from build123d import *

# Parameters (mm, degrees)
SKETCH2_R                             = 14
SKETCH2_R_2                           = 8
BOSS_EXTRUDE7_DEPTH                   = 15
SKETCH2_9_R                           = 16
SKETCH2_9_R_2                         = 13
BOSS_EXTRUDE8_DEPTH                   = 15
SKETCH2_11_R                          = 13
SKETCH2_11_R_2                        = 10
BOSS_EXTRUDE9_DEPTH                   = 9.5
BOSS_EXTRUDE11_REACH                  = 219.372
BOSS_EXTRUDE11_END_RADIUS             = 14
BOSS_EXTRUDE11_DIRECTION_2_REACH      = 219.372
BOSS_EXTRUDE11_DIRECTION_2_END_RADIUS = 16
BOSS_EXTRUDE12_REACH                  = 219.489
SKETCH15_W                            = 3
SKETCH15_H                            = 9.5
FILLET1_R                             = 2
SKETCH2_13_R                          = 8
SKETCH2_13_R_2                        = 4.25
BOSS_EXTRUDE13_DEPTH                  = 11


with BuildPart() as part:
    # Sketch2 → Boss-Extrude7 (new body)
    with BuildSketch(Plane(origin=(0, 0, 0), x_dir=(1, 0, 0), z_dir=(0, 1, 0))):
        with Locations(Location((-50, 3.220631283, 0), (0, 0, 270))):
            Circle(SKETCH2_R)
        with Locations(Location((-50, 3.220631283, 0), (0, 0, 270))):
            Circle(SKETCH2_R_2, mode=Mode.SUBTRACT)
    extrude(amount=BOSS_EXTRUDE7_DEPTH)


with BuildPart() as body_2:
    # Sketch2<9> → Boss-Extrude8 (new body)
    with BuildSketch(Plane(origin=(0, 0, 0), x_dir=(1, 0, 0), z_dir=(0, 1, 0))):
        with Locations(Location((200, 3.220631283, 0), (0, 0, 270))):
            Circle(SKETCH2_9_R)
        with Locations(Location((200, 3.220631283, 0), (0, 0, 270))):
            Circle(SKETCH2_9_R_2, mode=Mode.SUBTRACT)
    extrude(amount=BOSS_EXTRUDE8_DEPTH)

    # Sketch2<11> → Boss-Extrude9 (add)
    with BuildSketch(Plane(origin=(0, 0, 0), x_dir=(1, 0, 0), z_dir=(0, 1, 0))):
        with Locations(Location((200, 3.220631283, 0), (0, 0, 270))):
            Circle(SKETCH2_11_R)
        with Locations(Location((200, 3.220631283, 0), (0, 0, 270))):
            Circle(SKETCH2_11_R_2, mode=Mode.SUBTRACT)
    extrude(amount=BOSS_EXTRUDE9_DEPTH)


    add(part.part)  # Boss-Extrude11 merges part
    # Boss-Extrude11: up to this cylinder (the profile starts outside it)
    boss_extrude11_end = Plane(origin=(-50, 0.212132, -3.220631283), z_dir=(0, -1, 0)) * Cylinder(BOSS_EXTRUDE11_END_RADIUS, 467.744, mode=Mode.PRIVATE)
    # Sketch3 → Boss-Extrude11 (add, up to the surface)
    with BuildSketch(Plane(origin=(0, 0, 0), x_dir=(0, 0, -1), z_dir=(1, 0, 0)), mode=Mode.PRIVATE) as boss_extrude11_sk1:
        Polygon((10.720631283, 0), (10.720631283, 15), (-4.279368717, 15), (-4.279368717, 0), (-1.279368717, 0), (-1.279368717, 12), (7.720631283, 12), (7.720631283, 0), align=None)
    boss_extrude11_tool1 = extrude(boss_extrude11_sk1.sketch, amount=-BOSS_EXTRUDE11_REACH, mode=Mode.PRIVATE) - boss_extrude11_end
    add(boss_extrude11_tool1.solids().sort_by_distance((0, 0.212132, -9.220631))[0])

    # Boss-Extrude11 direction 2: up to this cylinder (the profile starts outside it)
    boss_extrude11_direction_2_end = Plane(origin=(200, 0.212132, -3.220631283), z_dir=(0, -1, 0)) * Cylinder(BOSS_EXTRUDE11_DIRECTION_2_END_RADIUS, 471.744, mode=Mode.PRIVATE)
    # Sketch3 → Boss-Extrude11 direction 2 (add, up to the surface)
    with BuildSketch(Plane(origin=(0, 0, 0), x_dir=(0, 0, -1), z_dir=(1, 0, 0)), mode=Mode.PRIVATE) as boss_extrude11_direction_2_sk1:
        Polygon((10.720631283, 0), (10.720631283, 15), (-4.279368717, 15), (-4.279368717, 0), (-1.279368717, 0), (-1.279368717, 12), (7.720631283, 12), (7.720631283, 0), align=None)
    boss_extrude11_direction_2_tool1 = extrude(boss_extrude11_direction_2_sk1.sketch, amount=BOSS_EXTRUDE11_DIRECTION_2_REACH, mode=Mode.PRIVATE) - boss_extrude11_direction_2_end
    add(boss_extrude11_direction_2_tool1.solids().sort_by_distance((0, 0.212132, -9.220631))[0])

    # Sketch15 → Boss-Extrude12 (add, up to next)
    with BuildSketch(Plane.XY.offset(-7.720631283), mode=Mode.PRIVATE) as boss_extrude12_sk1:
        with Locations((-14.45117452, 7.25)):
            Rectangle(SKETCH15_W, SKETCH15_H)
    boss_extrude12_tool1 = extrude(boss_extrude12_sk1.sketch, amount=BOSS_EXTRUDE12_REACH, mode=Mode.PRIVATE) - body_2.part
    # Sketch15 → Boss-Extrude12 (add, up to next)
    with BuildSketch(Plane.XY.offset(-7.720631283), mode=Mode.PRIVATE) as boss_extrude12_sk2:
        with Locations((86.457765729, 7.25)):
            Rectangle(SKETCH15_W, SKETCH15_H)
    boss_extrude12_tool2 = extrude(boss_extrude12_sk2.sketch, amount=BOSS_EXTRUDE12_REACH, mode=Mode.PRIVATE) - body_2.part
    # Sketch15 → Boss-Extrude12 (add, up to next)
    with BuildSketch(Plane.XY.offset(-7.720631283), mode=Mode.PRIVATE) as boss_extrude12_sk3:
        with Locations((10.776060542, 7.25)):
            Rectangle(SKETCH15_W, SKETCH15_H)
    boss_extrude12_tool3 = extrude(boss_extrude12_sk3.sketch, amount=BOSS_EXTRUDE12_REACH, mode=Mode.PRIVATE) - body_2.part
    # Sketch15 → Boss-Extrude12 (add, up to next)
    with BuildSketch(Plane.XY.offset(-7.720631283), mode=Mode.PRIVATE) as boss_extrude12_sk4:
        with Locations((36.003295604, 7.25)):
            Rectangle(SKETCH15_W, SKETCH15_H)
    boss_extrude12_tool4 = extrude(boss_extrude12_sk4.sketch, amount=BOSS_EXTRUDE12_REACH, mode=Mode.PRIVATE) - body_2.part
    # Sketch15 → Boss-Extrude12 (add, up to next)
    with BuildSketch(Plane.XY.offset(-7.720631283), mode=Mode.PRIVATE) as boss_extrude12_sk5:
        with Locations((61.230530666, 7.25)):
            Rectangle(SKETCH15_W, SKETCH15_H)
    boss_extrude12_tool5 = extrude(boss_extrude12_sk5.sketch, amount=BOSS_EXTRUDE12_REACH, mode=Mode.PRIVATE) - body_2.part
    # Sketch15 → Boss-Extrude12 (add, up to next)
    with BuildSketch(Plane.XY.offset(-7.720631283), mode=Mode.PRIVATE) as boss_extrude12_sk6:
        with Locations((111.685000791, 7.25)):
            Rectangle(SKETCH15_W, SKETCH15_H)
    boss_extrude12_tool6 = extrude(boss_extrude12_sk6.sketch, amount=BOSS_EXTRUDE12_REACH, mode=Mode.PRIVATE) - body_2.part
    # Sketch15 → Boss-Extrude12 (add, up to next)
    with BuildSketch(Plane.XY.offset(-7.720631283), mode=Mode.PRIVATE) as boss_extrude12_sk7:
        with Locations((136.912235853, 7.25)):
            Rectangle(SKETCH15_W, SKETCH15_H)
    boss_extrude12_tool7 = extrude(boss_extrude12_sk7.sketch, amount=BOSS_EXTRUDE12_REACH, mode=Mode.PRIVATE) - body_2.part
    # Sketch15 → Boss-Extrude12 (add, up to next)
    with BuildSketch(Plane.XY.offset(-7.720631283), mode=Mode.PRIVATE) as boss_extrude12_sk8:
        with Locations((162.139470915, 7.25)):
            Rectangle(SKETCH15_W, SKETCH15_H)
    boss_extrude12_tool8 = extrude(boss_extrude12_sk8.sketch, amount=BOSS_EXTRUDE12_REACH, mode=Mode.PRIVATE) - body_2.part
    add(boss_extrude12_tool1.solids().sort_by_distance((-14.451175, 7.25, -7.720631))[0])
    add(boss_extrude12_tool2.solids().sort_by_distance((86.457766, 7.25, -7.720631))[0])
    add(boss_extrude12_tool3.solids().sort_by_distance((10.776061, 7.25, -7.720631))[0])
    add(boss_extrude12_tool4.solids().sort_by_distance((36.003296, 7.25, -7.720631))[0])
    add(boss_extrude12_tool5.solids().sort_by_distance((61.230531, 7.25, -7.720631))[0])
    add(boss_extrude12_tool6.solids().sort_by_distance((111.685001, 7.25, -7.720631))[0])
    add(boss_extrude12_tool7.solids().sort_by_distance((136.912236, 7.25, -7.720631))[0])
    add(boss_extrude12_tool8.solids().sort_by_distance((162.139471, 7.25, -7.720631))[0])

    # Fillet1
    fillet1_edges = [body_2.edges().sort_by_distance(p)[0] for p in [
        (59.730530666, 7.25, 1.279368717),
        (62.730530666, 7.25, 1.279368717),
        (62.730530666, 7.25, -7.720631283),
        (59.730530666, 7.25, -7.720631283),
        (110.185000791, 7.25, 1.279368717),
        (113.185000791, 7.25, 1.279368717),
        (113.185000791, 7.25, -7.720631283),
        (110.185000791, 7.25, -7.720631283),
        (135.412235853, 7.25, 1.279368717),
        (138.412235853, 7.25, 1.279368717),
        (138.412235853, 7.25, -7.720631283),
        (135.412235853, 7.25, -7.720631283),
        (160.639470915, 7.25, 1.279368717),
        (163.639470915, 7.25, 1.279368717),
        (163.639470915, 7.25, -7.720631283),
        (160.639470915, 7.25, -7.720631283),
        (-15.95117452, 7.25, 1.279368717),
        (-12.95117452, 7.25, 1.279368717),
        (-12.95117452, 7.25, -7.720631283),
        (-15.95117452, 7.25, -7.720631283),
        (84.957765729, 7.25, 1.279368717),
        (87.957765729, 7.25, 1.279368717),
        (87.957765729, 7.25, -7.720631283),
        (84.957765729, 7.25, -7.720631283),
        (12.276060542, 7.25, 1.279368717),
        (9.276060542, 7.25, 1.279368717),
        (12.276060542, 7.25, -7.720631283),
        (9.276060542, 7.25, -7.720631283),
        (34.503295604, 7.25, 1.279368717),
        (37.503295604, 7.25, 1.279368717),
        (37.503295604, 7.25, -7.720631283),
        (34.503295604, 7.25, -7.720631283),
    ]]
    fillet(fillet1_edges, radius=FILLET1_R)

    # Sketch2<13> → Boss-Extrude13 (add)
    with BuildSketch(Plane(origin=(0, 0, 0), x_dir=(1, 0, 0), z_dir=(0, 1, 0))):
        with Locations(Location((-50, 3.220631283, 0), (0, 0, 270))):
            Circle(SKETCH2_13_R)
        with Locations(Location((-50, 3.220631283, 0), (0, 0, 270))):
            Circle(SKETCH2_13_R_2, mode=Mode.SUBTRACT)
    extrude(amount=BOSS_EXTRUDE13_DEPTH)


solid = body_2.part
Geometry: final body of the model. Coordinates: model frame, mm. A direction names the side the tool comes from. Coordinates: 2 decimals unless noted, no trailing zeros. Order: outer loops, then holes, each group sorted by start corner. A loop starts at its lowest first (then second) coordinate and runs counter-clockwise, first axis right, second up.
(1) Material intervals for probe 1 along Z at (x, y) = (94, 3.75); probe 2 along Y at (x, z) = (-4.5, -7.5); probe 3 along X at (y, z) = (5.25, 6), sorted ascending.
(2) Access query for faces 1 (the face through (190.24, 4.68, -5.39)), 2 (the face through (72, 7, -10.721)), 3 (the face through (99, 12, -3)). Directions: +Z, -Z, +X, -X, +Y, -Y. A direction counts if a zero-diameter tool reaches every point of the face in a straight line with its end or side. Return the directions, or none.
(3) Section query B-B (x = 200). Return the cut outline in (y, z), plus the area to 3 significant figures.
(4) Section query C-C (x = 170). Return the cut outline in (y, z), plus the area to 3 significant figures.
(5) Section query A-A (x = -50). Return the cut outline in (y, z), plus the area to 4 significant figures.
(6) First-contact query: pin 1 (6 mm diameter, centred on x = 91.5, y = 5, fed in from -Z); pin 2 (1.5 mm diameter, centred on y = 9.5, z = -2, fed in from +X); pin 3 (3.5 mm diameter, centred on x = 163.5, z = -4.5, fed in from -Y). Flat tips, straight axial feed; report the tip coordinate or a pass-through.
(7) Section query D-D (y = 5.25). State how many separate pieces and enclosed holes the cut face has, plus the area to 3 significant figures.
(8) Draft query along X for faces 4 (the face through (74, 15, -3)), 5 (the face through (174, 12, -3)). Return one class per face: pulls with the +X half, pulls with the -X half, needs draft (parallel to the pull), parting line crosses it, or undercut.
Solution:
1. probe 1: z = -10.72 to -7.72, 1.28 to 4.28
1. probe 2: y = 12 to 15
1. probe 3: x = -60.53 to -39.47, 186.92 to 196.13, 203.87 to 213.08
2. face 1: +Y, -Y
2. face 2: -Z, +Y, -Y
2. face 3: -Y
3. outline: (0, -19.22) - (15, -19.22) - (15, -16.22) - (9.5, -16.22) - (9.5, -13.22) - (0, -13.22) - close; (0, 6.78) - (9.5, 6.78) - (9.5, 9.78) - (15, 9.78) - (15, 12.78) - (0, 12.78) - close
3. area: 147 mm2
4. outline: (0, -10.72) - (15, -10.72) - (15, 4.28) - (0, 4.28) - (0, 1.28) - (12, 1.28) - (12, -7.72) - (0, -7.72) - close
4. area: 117 mm2
5. outline: (0, -17.22) - (15, -17.22) - (15, -11.22) - (11, -11.22) - (11, -7.47) - (0, -7.47) - close; (0, 1.03) - (11, 1.03) - (11, 4.78) - (15, 4.78) - (15, 10.78) - (0, 10.78) - close
5. area: 262.5 mm2
6. pin 1: stops at z = -10.72
6. pin 2: stops at x = 215.99
6. pin 3: stops at y = 2.5
7. separate pieces: 1
7. enclosed holes: 11
7. area: 2,630 mm2
8. face 4: needs draft
8. face 5: undercut
